Design review of the part shown in the three views and the two pictorial views. Dimensions are in mm from the part's minimum x, y and z. Coordinates: 2 decimals unless noted, no trailing zeros. Write each loop counter-clockwise with the first axis right and the second up, starting at its lowest first coordinate (ties: lowest second). Pieces come first, ordered by that corner, then holes.
Q1. Take a section at C-C, the plane z = 20. Write out the cut boundary in (x, y) (3 decimals), plus the area to 3 significant figures.
Q2. Take a section at D-D, the plane x = 75. Write out the cut boundary in (y, z) (3 decimals).
Q3. The part is to be moulded in two halves that separate along X. For the marked faces 1 and 2, say which applies: released by +X, released by -X, zero draft, split by the parting line, or undercut.
Q4. For L1, parallel to X at y = 13, z = 11; L2, parallel to X at y = 13.5, z = 16.5; L3, parallel to Z at x = 84.5, y = 4.25, list the stretches that pass through material, from the lowest coordinate up.
Q5. For pin 1 Ø1 at (y, z) = (9, 14.5) entering from +X; pin 2 Ø6 at (y, z) = (14, 8.5) entering from -X; pin 3 Ø17 at (x, z) = (22, 22) entering from +Y; pin 4 Ø1.5 at (x, y) = (84.5, 7.5) entering from +Z, all flat-tipped, find the tip position at first contact; note any pin that passes through.
Q6. Take a section at B-B, the plane y = 7.5. Write out the cut boundary in (x, z) (1 decimal), plus the area to 3 significant figures.
Q7. Take a section at A-A, the plane x = 34.5. Write out the cut boundary in (y, z) (3 decimals).
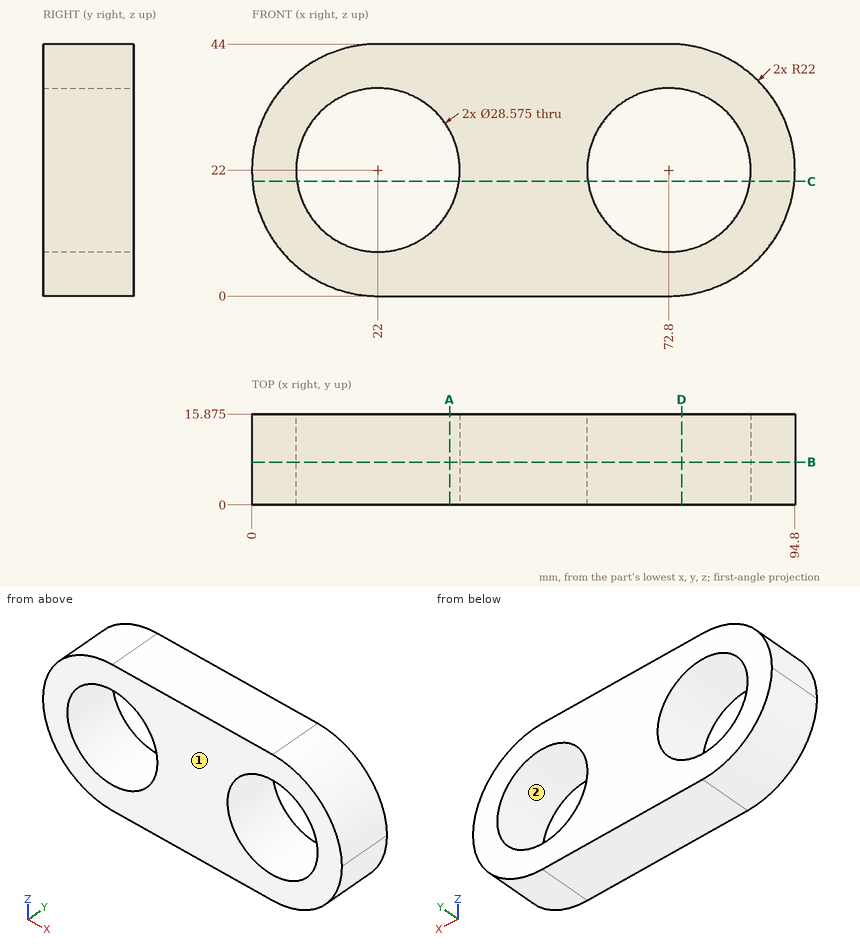
Responses:
1. outline: (0.091, 0) - (7.853, 0) - (7.853, 15.875) - (0.091, 15.875) - close; (36.147, 0) - (58.653, 0) - (58.653, 15.875) - (36.147, 15.875) - close; (86.947, 0) - (94.709, 0) - (94.709, 15.875) - (86.947, 15.875) - close
1. area: 604 mm2
2. outline: (0, 0.11) - (15.875, 0.11) - (15.875, 7.883) - (0, 7.883) - close; (0, 36.117) - (15.875, 36.117) - (15.875, 43.89) - (0, 43.89) - close
3. face 1: zero draft
3. face 2: undercut
4. L1: x = 2.95 to 12.88, 31.12 to 63.68, 81.92 to 91.85
4. L2: x = 0.7 to 8.81, 35.19 to 59.61, 85.99 to 94.1
4. L3: z = 3.37 to 13.8, 30.2 to 40.63
5. pin 1: stops at x = 93.66
5. pin 2: stops at x = 2.67
5. pin 3: passes through
5. pin 4: stops at z = 41.08
6. outline: (22, 0) - (72.8, 0) arc R22 ccw to (72.8, 44) - (22, 44) arc R22 ccw to start; hole circle Ø28.6 at (22, 22); hole circle Ø28.6 at (72.8, 22)
6. area: 2,470 mm2
7. outline: (0, 0) - (15.875, 0) - (15.875, 15.08) - (0, 15.08) - close; (0, 28.92) - (15.875, 28.92) - (15.875, 44) - (0, 44) - close
